Work out the finished part from the listing and answer in its coordinate system (mm). Coordinates: 2 decimals unless noted, no trailing zeros. Write each loop counter-clockwise with the first axis right and the second up, starting at its lowest first coordinate (ties: lowest second). Pieces come first, ordered by that corner, then holes. Notation, with made-up numbers: (75, 20.5) - (120, 20.5) arc R13 ccw to (120, 25.5) - close; hole circle Ø5 at (73.5, -12). An arc over 180 degrees is marked (long way). One line per item, written item: value.
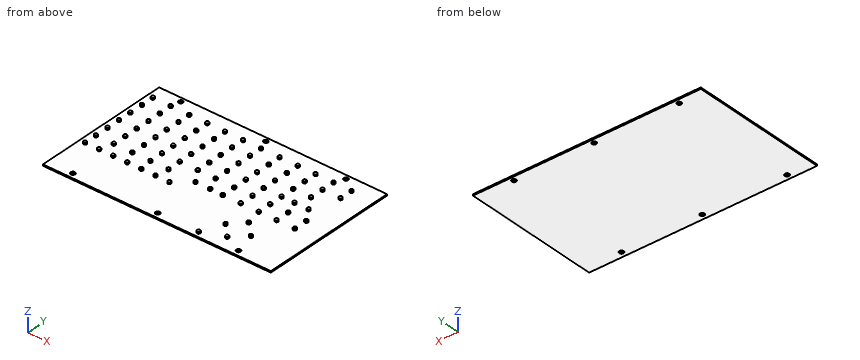
```python
from build123d import *

# Parameters (mm, degrees)
SKETCH_2_W          = 129.667
SKETCH_2_H          = 78.613
EXTRUDE_1_DEPTH     = 0.8
SKETCH_3_R          = 1.27
CUT_EXTRUDE_1_DEPTH = 12.54
SKETCH_4_R          = 0.92202
SKETCH_4_R_2        = 0.922029104
SKETCH_4_R_3        = 0.919681264
SKETCH_4_R_4        = 0.924963229
SKETCH_4_R_5        = 0.92552898
EXTRUDE_2_DEPTH     = 1


with BuildPart() as part:
    # 草图2 → 凸台-拉伸1 (new body)
    with BuildSketch(Plane.XY):
        with Locations((83.3755, 41.2115)):
            Rectangle(SKETCH_2_W, SKETCH_2_H)
    extrude(amount=EXTRUDE_1_DEPTH)

    # 草图3 → 切除-拉伸1 (cut)
    with BuildSketch(Plane.XY.offset(0.8)):
        with Locations((33.02, 77.978)):
            Circle(SKETCH_3_R)
        with Locations((81.28, 78.105)):
            Circle(SKETCH_3_R)
        with Locations((127, 77.978)):
            Circle(SKETCH_3_R)
        with Locations((33.02, 4.953)):
            Circle(SKETCH_3_R)
        with Locations((81.28, 4.953)):
            Circle(SKETCH_3_R)
        with Locations((127.127, 5.08)):
            Circle(SKETCH_3_R)
    extrude(amount=-CUT_EXTRUDE_1_DEPTH, mode=Mode.SUBTRACT)

    # 草图4 → 凸台-拉伸2 (add)
    with BuildSketch(Plane.XY.offset(0.8)):
        with Locations((22.098, 72.009)):
            Circle(SKETCH_4_R)
        with Locations((22.098, 64.643)):
            Circle(SKETCH_4_R)
        with Locations((22.098, 56.769)):
            Circle(SKETCH_4_R)
        with Locations((22.098, 49.149)):
            Circle(SKETCH_4_R)
        with Locations((22.098, 26.162)):
            Circle(SKETCH_4_R)
        with Locations((22.098, 33.528)):
            Circle(SKETCH_4_R)
        with Locations((22.098, 41.275)):
            Circle(SKETCH_4_R)
        with Locations((32.258, 72.009)):
            Circle(SKETCH_4_R)
        with Locations((42.926, 71.882)):
            Circle(SKETCH_4_R)
        with Locations((53.086, 72.009)):
            Circle(SKETCH_4_R)
        with Locations((63.246, 71.882)):
            Circle(SKETCH_4_R)
        with Locations((73.533, 71.882)):
            Circle(SKETCH_4_R)
        with Locations((83.693, 71.882)):
            Circle(SKETCH_4_R)
        with Locations((94.361, 71.882)):
            Circle(SKETCH_4_R)
        with Locations((104.648, 71.882)):
            Circle(SKETCH_4_R)
        with Locations((114.808, 71.882)):
            Circle(SKETCH_4_R)
        with Locations((124.968, 71.882)):
            Circle(SKETCH_4_R)
        with Locations((135.255, 71.882)):
            Circle(SKETCH_4_R)
        with Locations((32.385, 64.516)):
            Circle(SKETCH_4_R)
        with Locations((32.385, 56.769)):
            Circle(SKETCH_4_R)
        with Locations((32.258, 49.022)):
            Circle(SKETCH_4_R)
        with Locations((32.258, 33.528)):
            Circle(SKETCH_4_R)
        with Locations((32.258, 41.275)):
            Circle(SKETCH_4_R)
        with Locations((54.102, 26.162)):
            Circle(SKETCH_4_R)
        with Locations((30.099, 26.162)):
            Circle(SKETCH_4_R)
        with Locations((38.1, 26.162)):
            Circle(SKETCH_4_R)
        with Locations((46.101, 26.162)):
            Circle(SKETCH_4_R)
        with Locations((42.926, 64.643)):
            Circle(SKETCH_4_R)
        with Locations((42.799, 56.769)):
            Circle(SKETCH_4_R)
        with Locations((53.086, 64.516)):
            Circle(SKETCH_4_R)
        with Locations((63.246, 64.516)):
            Circle(SKETCH_4_R)
        with Locations((53.086, 56.769)):
            Circle(SKETCH_4_R)
        with Locations((63.246, 56.769)):
            Circle(SKETCH_4_R)
        with Locations((42.937232377, 49.080669284)):
            Circle(SKETCH_4_R)
        with Locations((53.086, 49.022)):
            Circle(SKETCH_4_R)
        with Locations((63.246, 49.022)):
            Circle(SKETCH_4_R)
        with Locations((42.927878215, 41.278345649)):
            Circle(SKETCH_4_R)
        with Locations((42.78999374, 33.521368778)):
            Circle(SKETCH_4_R)
        with Locations((53.086, 33.528)):
            Circle(SKETCH_4_R)
        with Locations((53.096022403, 41.290450758)):
            Circle(SKETCH_4_R)
        with Locations((104.775, 4.699)):
            Circle(SKETCH_4_R)
        with Locations((116.84, 9.652)):
            Circle(SKETCH_4_R_2)
        with Locations((109.855, 16.891)):
            Circle(SKETCH_4_R)
        with Locations((124.333, 16.764)):
            Circle(SKETCH_4_R_3)
        with Locations((116.84, 24.257)):
            Circle(SKETCH_4_R_4)
        with Locations((135.255, 33.528)):
            Circle(SKETCH_4_R_5)
        with Locations((135.255, 41.275)):
            Circle(SKETCH_4_R)
        with Locations((124.968, 33.401)):
            Circle(SKETCH_4_R)
        with Locations((124.968, 41.275)):
            Circle(SKETCH_4_R)
        with Locations((114.808, 33.401)):
            Circle(SKETCH_4_R)
        with Locations((114.808, 41.148)):
            Circle(SKETCH_4_R)
        with Locations((130.175, 48.895)):
            Circle(SKETCH_4_R)
        with Locations((122.174, 48.895)):
            Circle(SKETCH_4_R)
        with Locations((114.808, 48.895)):
            Circle(SKETCH_4_R)
        with Locations((124.968, 56.769)):
            Circle(SKETCH_4_R)
        with Locations((114.808, 56.769)):
            Circle(SKETCH_4_R)
        with Locations((114.808, 64.516)):
            Circle(SKETCH_4_R)
        with Locations((124.968, 64.516)):
            Circle(SKETCH_4_R)
        with Locations((135.255, 64.516)):
            Circle(SKETCH_4_R)
        with Locations((62.103, 26.162)):
            Circle(SKETCH_4_R)
        with Locations((70.104, 26.162)):
            Circle(SKETCH_4_R)
        with Locations((63.373, 33.528)):
            Circle(SKETCH_4_R)
        with Locations((78.74, 33.528)):
            Circle(SKETCH_4_R)
        with Locations((87.122, 33.528)):
            Circle(SKETCH_4_R)
        with Locations((104.521, 33.528)):
            Circle(SKETCH_4_R)
        with Locations((94.361, 33.401)):
            Circle(SKETCH_4_R)
        with Locations((73.533, 41.275)):
            Circle(SKETCH_4_R)
        with Locations((63.246, 41.275)):
            Circle(SKETCH_4_R)
        with Locations((83.693, 41.275)):
            Circle(SKETCH_4_R)
        with Locations((104.648, 41.275)):
            Circle(SKETCH_4_R)
        with Locations((94.361, 41.148)):
            Circle(SKETCH_4_R)
        with Locations((73.533, 49.022)):
            Circle(SKETCH_4_R)
        with Locations((83.693, 49.022)):
            Circle(SKETCH_4_R)
        with Locations((94.361, 49.022)):
            Circle(SKETCH_4_R)
        with Locations((104.521, 49.022)):
            Circle(SKETCH_4_R)
        with Locations((73.533, 64.516)):
            Circle(SKETCH_4_R)
        with Locations((73.533, 56.769)):
            Circle(SKETCH_4_R)
        with Locations((83.693, 64.516)):
            Circle(SKETCH_4_R)
        with Locations((83.693, 56.769)):
            Circle(SKETCH_4_R)
        with Locations((94.361, 64.516)):
            Circle(SKETCH_4_R)
        with Locations((94.361, 56.642)):
            Circle(SKETCH_4_R)
        with Locations((104.521, 56.642)):
            Circle(SKETCH_4_R)
        with Locations((104.648, 64.516)):
            Circle(SKETCH_4_R)
    extrude(amount=EXTRUDE_2_DEPTH)


solid = part.part
```
Item 1: Section A-A, the plane x = 81.28 is taken. Determine the outline of the cut face in (y, z) (3 decimals).
Evaluation:
outline: (1.905, 0) - (3.683, 0) - (3.683, 0.8) - (1.905, 0.8) - close; (6.223, 0) - (76.835, 0) - (76.835, 0.8) - (6.223, 0.8) - close; (79.375, 0) - (80.518, 0) - (80.518, 0.8) - (79.375, 0.8) - close
Item 2: Given pin 1 (4 mm diameter, centred on x = 86, y = 39, fed in from +Z), flat-ended and moving along its own axis, determine where the tip first touches the part or whether it passes through.
Evaluation:
pin 1: stops at z = 0.8
Item 3: Section C-C, the plane x = 139.5 is taken. Determine the outline of the cut face in (y, z) (3 decimals).
Evaluation:
outline: (1.905, 0) - (80.518, 0) - (80.518, 0.8) - (1.905, 0.8) - close
Item 4: Consider probe 1 along Y at (x, z) = (81.28, 0.3) (3 decimals); probe 2 along Y at (x, z) = (127, 0.2) (3 decimals); probe 3 along Z at (x, y) = (27, 74). Determine where each line is inside the solid, lowest interval first.
Evaluation:
probe 1: y = 1.905 to 3.683, 6.223 to 76.835, 79.375 to 80.518
probe 2: y = 1.905 to 3.816, 6.344 to 76.708, 79.248 to 80.518
probe 3: z = 0 to 0.8
Item 5: Section B-B, the plane y = 19.5 is taken. Determine the outline of the cut face in (x, z).
Evaluation:
outline: (18.54, 0) - (148.21, 0) - (148.21, 0.8) - (18.54, 0.8) - close
